The listing builds one solid part. Answer for the finished solid, in the listing's coordinates (mm). Face numbers are marked on the shaded views. A direction names the side the tool comes from. Round coordinates to 2 decimals unless told otherwise and drop trailing zeros. Write each loop counter-clockwise with the first axis right and the second up, starting at its lowest first coordinate (ties: lowest second). Pieces come first, ordered by that corner, then holes.
Item 1: Find section A-A on z = 0. Give the vertices of the cut face in (x, y).
Item 2: Find section B-B on x = -39. Give the vertices of the cut face in (y, z), then the cut area to 3 significant figures.
Item 3: A tool of negligible diameter and unlimited length cuts with its end or side. For the marked faces 1 and 2, from which of +Z, -Z, +X, -X, +Y, -Y can it reach the whole face along a straight path? Write none if from no direction.
Item 4: For a pull along X with two mould halves and no side action, classify the marked faces 3 and 4 as +X half, -X half, draft (parallel to the pull), parting line (faces both ways), or undercut.
Item 5: Each of these flat-tipped pins is pushed along its axis until it touches: pin 1 (6 mm diameter, centred on y = 2, z = -5.5, fed in from -X); pin 2 (7.5 mm diameter, centred on x = -37.5, z = 0, fed in from -Y); pin 3 (7.5 mm diameter, centred on x = 35.5, z = -0.5, fed in from +Y); pin 4 (4 mm diameter, centred on y = 8, z = 1, fed in from +X). Where does it stop, or does it pass through?
Item 6: Find section D-D on y = 6.5. Give the vertices of the cut face in (x, z), then the cut area to 3 significant figures.
Item 7: Find the intervals of material crossed by probe 1 along X at (y, z) = (1.4, 0); probe 2 along X at (y, z) = (8.5, 0); probe 3 along Y at (x, z) = (-37.5, -4.25), in increasing order.
Item 8: Find section C-C on z = 6. Give the vertices of the cut face in (x, y).
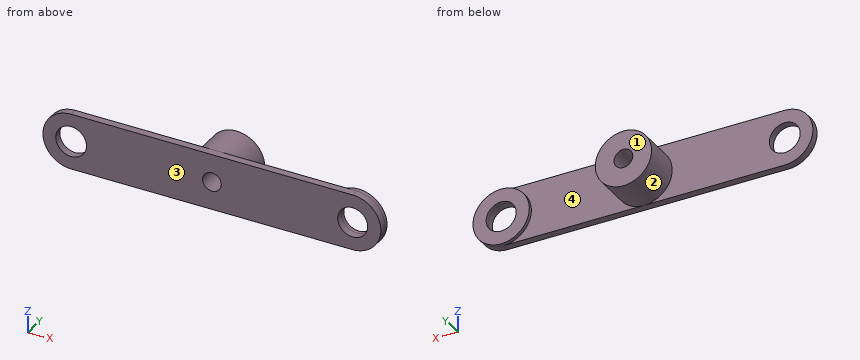
```python
from build123d import *
from build123d.topology import SkipClean

# Parameters (mm, degrees)
SKETCH1_R           = 4.1
SKETCH1_R_2         = 4
BOSS_EXTRUDE1_DEPTH = 2
SKETCH3_R           = 7.5
BOSS_EXTRUDE3_DEPTH = 10
SKETCH4_R           = 2.5
CUT_EXTRUDE1_DEPTH  = 48.172555581
SKETCH5_R           = 7.5
SKETCH5_R_2         = 4
BOSS_EXTRUDE4_DEPTH = 1


with BuildPart() as part:
    # Sketch1 → Boss-Extrude1 (new body)
    with BuildSketch(Plane(origin=(0, 0, 0), x_dir=(1, 0, 0), z_dir=(0, 1, 0))):
        with BuildLine():
            Line((-37.5, 7.5), (37.5, 7.5))
            ThreePointArc((37.5, 7.5), (45, 0), (37.5, -7.5))
            Line((37.5, -7.5), (-37.5, -7.5))
            ThreePointArc((-37.5, -7.5), (-45, 0), (-37.5, 7.5))
        make_face()
        with Locations(Location((-37.5, 0, 0), (0, 0, 270))):
            Circle(SKETCH1_R, mode=Mode.SUBTRACT)
        with Locations(Location((37.5, 0, 0), (0, 0, 270))):
            Circle(SKETCH1_R_2, mode=Mode.SUBTRACT)
    extrude(amount=BOSS_EXTRUDE1_DEPTH)

    # Sketch3 → Boss-Extrude3 (add)
    with BuildSketch(Plane(origin=(0, 2, 0), x_dir=(1, 0, 0), z_dir=(0, 1, 0))):
        with Locations(Location((0, 0, 0), (0, 0, 270))):
            Circle(SKETCH3_R)
    extrude(amount=BOSS_EXTRUDE3_DEPTH)

    # Sketch4 → Cut-Extrude1 (cut, through all)
    with BuildSketch(Plane(origin=(0, 12, 0), x_dir=(1, 0, 0), z_dir=(0, 1, 0))):
        with Locations(Location((0, 0, 0), (0, 0, 270))):
            Circle(SKETCH4_R)
    extrude(amount=-CUT_EXTRUDE1_DEPTH, mode=Mode.SUBTRACT)

    # Sketch5 → Boss-Extrude4 (add)
    with SkipClean():  # the faces are left unmerged after this step: merging them gives an invalid solid
        with BuildSketch(Plane(origin=(0, 2, 0), x_dir=(1, 0, 0), z_dir=(0, 1, 0))):
            with Locations(Location((37.5, 0, 0), (0, 0, 270))):
                Circle(SKETCH5_R)
            with Locations(Location((37.5, 0, 0), (0, 0, 270))):
                Circle(SKETCH5_R_2, mode=Mode.SUBTRACT)
        extrude(amount=BOSS_EXTRUDE4_DEPTH)
    add(part.part.scale(1), mode=Mode.REPLACE)  # the faces are merged on a copy


solid = part.part
```
Check values:
1. outline: (-45, 0) - (-41.6, 0) - (-41.6, 2) - (-45, 2) - close; (-33.4, 0) - (-2.5, 0) - (-2.5, 12) - (-7.5, 12) - (-7.5, 2) - (-33.4, 2) - close; (2.5, 0) - (33.5, 0) - (33.5, 3) - (30, 3) - (30, 2) - (7.5, 2) - (7.5, 12) - (2.5, 12) - close; (41.5, 0) - (45, 0) - (45, 3) - (41.5, 3) - close
2. outline: (0, -7.35) - (2, -7.35) - (2, -3.82) - (0, -3.82) - close; (0, 3.82) - (2, 3.82) - (2, 7.35) - (0, 7.35) - close
2. area: 14.1 mm2
3. face 1: +Z, -Z, +X, -X, +Y
3. face 2: +Y
4. face 3: draft
4. face 4: undercut
5. pin 1: stops at x = -44.57
5. pin 2: passes through
5. pin 3: stops at y = 3
5. pin 4: stops at x = 7.5
6. outline: circle Ø15 at (0, 0); hole circle Ø5 at (0, 0)
6. area: 157 mm2
7. probe 1: x = -45 to -41.6, -33.4 to -2.5, 2.5 to 33.5, 41.5 to 45
7. probe 2: x = -7.5 to -2.5, 2.5 to 7.5
7. probe 3: y = 0 to 2
8. outline: (-42, 0) - (42, 0) - (42, 3) - (33, 3) - (33, 2) - (4.5, 2) - (4.5, 12) - (-4.5, 12) - (-4.5, 2) - (-42, 2) - close
